Autodesk Inventor part; units mm, degrees
ref_plane "YZ Plane" through (0, 0, 0) normal (1, 0, 0) x (0, 1, 0)
ref_plane "XZ Plane" through (0, 0, 0) normal (0, 1, 0) x (-1, 0, 0)
ref_plane "XY Plane" through (0, 0, 0) normal (0, 0, 1) x (1, 0, 0)
sketch "Sketch1" plane through (0, 0, 0) normal (1, 0, 0) x (0, 1, 0)
  circle A0 centre (0, 0) radius 35
  dimension "d0" = 70
extrude "Extrusion1" add sketch "Sketch1" along normal blind 50
sketch "Sketch2" plane through (50, 0, 0) normal (1, 0, 0) x (0, 0, -1)
  circle A0 centre (0, 0) radius 42.5
  dimension "d3" = 85
extrude "Extrusion2" add sketch "Sketch2" along normal blind 40
sketch "Sketch3" plane through (90, 0, 0) normal (1, 0, 0) x (0, 0, -1)
  line L0 (0, 30.5873) -> (26.4894, 15.2937)
  line L1 (26.4894, 15.2937) -> (26.4894, -15.2937)
  line L2 (26.4894, -15.2937) -> (0, -30.5873)
  line L3 (0, -30.5873) -> (-26.4894, -15.2937)
  line L4 (-26.4894, -15.2937) -> (-26.4894, 15.2937)
  line L5 (-26.4894, 15.2937) -> (0, 30.5873)
  point P0 (0, 0)
  point P1 (0, 0)
extrude "Extrusion3" add sketch "Sketch3" along normal blind 20
sketch "Sketch4" plane through (110, 0, 0) normal (1, 0, 0) x (0, 0, -1)
  circle A0 centre (0, 0) radius 12.5
  dimension "d8" = 25
extrude "Extrusion4" add sketch "Sketch4" along normal blind 3
sketch "Sketch5" plane through (113, 0, 0) normal (1, 0, 0) x (0, 0, -1)
  circle A0 centre (0, 0) radius 12.0251
extrude "Extrusion5" add sketch "Sketch5" along normal blind 3
sketch "Sketch6" plane through (116, 0, 0) normal (1, 0, 0) x (0, 0, -1)
  circle A0 centre (0, 0) radius 11.5831
extrude "Extrusion6" add sketch "Sketch6" along normal blind 3
sketch "Sketch7" plane through (119, 0, 0) normal (1, 0, 0) x (0, 0, -1)
  circle A0 centre (0, 0) radius 4.75
  dimension "d16" = 9.5
extrude "Extrusion7" add sketch "Sketch7" along normal blind 60
sketch "Sketch8" plane through (0, 0, 0) normal (0, 1, 0) x (-1, 0, 0)
  circle A0 centre (-136.5365, 0) radius 1.25
  point P0 (0, 0)
  dimension "d19" = 2.5
extrude "Extrusion8" cut sketch "Sketch8" along normal mid plane 20
properties part number "DC" material "Aluminum 6061-AHC"
The listing builds one solid part. Answer for the finished solid, in the listing's coordinates (mm). A direction names the side the tool comes from. Coordinates: 2 decimals unless noted, no trailing zeros. Write each loop counter-clockwise with the first axis right and the second up, starting at its lowest first coordinate (ties: lowest second). Pieces come first, ordered by that corner, then holes. Notation, with made-up numbers: (28.5, 27.5) -> (48.5, 27.5) arc R15 ccw to (48.5, 35.5) -> close; hole circle Ø5 at (11, 3.25). An arc over 180 degrees is marked (long way). Write each question's results on one line, items separated by ' | '. Start each with the question number.
1) A cutting plane is placed at C-C (x = 163). Determine the outline of the cut face in (y, z).
2) A tool of negligible diameter and unlimited length cuts with its end or side. For faces 1 (the flat face through (99.86, 22.833, 13.43)), 2 (the flat face through (90, 1, -28)), 3 (the flat face through (99.86, -22.833, -13.43)), from which of +Z, -Z, +X, -X, +Y, -Y can it reach the whole face along a straight path? Write none if from no direction.
3) Straight lines are drawn through the part: probe 1 along X at (y, z) = (-1.5, 0); probe 2 along X at (y, z) = (7.5, 0); probe 3 along X at (y, z) = (31, 12.5). For each, find the intervals that lie inside material, in ascending order.
4) A cutting plane is placed at B-B (y = 28). Determine the outline of the cut face in (x, z).
5) A cutting plane is placed at D-D (z = 9.5). Determine the outline of the cut face in (x, y).
6) Flat-ended cylindrical pins translate along their axes: pin 1 Ø12 at (x, z) = (155.5, -0.5) entering from +Y; pin 2 Ø12.5 at (y, z) = (1, 6) entering from +X; pin 3 Ø5 at (x, y) = (75.5, -4) entering from +Z; pin 4 Ø16 at (x, y) = (100.5, 0) entering from +Z. Find the tip coordinate at first contact, or state that the pin passes through.
Values follow:
1) outline: circle Ø9.5 at (0, 0)
2) face 1: +Z, +X, +Y | face 2: +X | face 3: -Z, +X, -Y
3) probe 1: 0 to 135.29, 137.79 to 179 | probe 2: 0 to 119 | probe 3: 0 to 90
4) outline: (0, -21) -> (50, -21) -> (50, -31.97) -> (90, -31.97) -> (90, -4.48) -> (110, -4.48) -> (110, 4.48) -> (90, 4.48) -> (90, 31.97) -> (50, 31.97) -> (50, 21) -> (0, 21) -> close
5) outline: (0, -33.69) -> (50, -33.69) -> (50, -41.42) -> (90, -41.42) -> (90, -25.1) -> (110, -25.1) -> (110, -8.12) -> (113, -8.12) -> (113, -7.37) -> (116, -7.37) -> (116, -6.63) -> (119, -6.63) -> (119, 6.63) -> (116, 6.63) -> (116, 7.37) -> (113, 7.37) -> (113, 8.12) -> (110, 8.12) -> (110, 25.1) -> (90, 25.1) -> (90, 41.42) -> (50, 41.42) -> (50, 33.69) -> (0, 33.69) -> close
6) pin 1: y = 4.75 | pin 2: x = 179 | pin 3: z = 42.47 | pin 4: z = 26.49
